Can you work these out from the model? Positions are in its coordinate system, mm. A direction names the side the tool comes from. Give positions to 0.01 mm unless a question says otherwise; leave off trailing zeros. Write each loop counter-clockwise with the first axis right and the second up, starting at its lowest first coordinate (ties: lowest second). Pieces come first, ordered by that corner, then holes. Notation, with made-up numbers: (-25.75, 10) - (15.25, 10) arc R22 cw to (15.25, 36) - close; hole circle Ø5 at (6, 24). An arc over 180 degrees is marked (long way). Return JSON: item names as keys, results as strings. Group by question number.
from build123d import *

# Parameters (mm, degrees)
F0_W      = 60
F0_H      = 60
F1_DEPTH  = 15
F2_W      = 25
F2_H      = 10
F3_DEPTH  = 150
F4_W      = 40
F4_H      = 40
F4_W_2    = 25
F4_H_2    = 10
F5_DEPTH  = 25
F6_SIZE2  = 39.99999
F6_SIZE   = 19.99999
F7_W      = 20
F7_H      = 5
F8_DEPTH  = 25
F9_R      = 3.5
F10_DEPTH = 150
F11_R     = 4
F12_DEPTH = 150


# Not quite as in the source:
# - a fillet or chamfer is up to 0.001 mm smaller than in the source, because OpenCascade refuses the exact size


with BuildPart() as f1:
    # F0 (on Top) → F1 (new body)
    with BuildSketch(Plane.XY):
        Rectangle(F0_W, F0_H)
    extrude(amount=F1_DEPTH)

    # F2 (on face) → F3 (join)
    with BuildSketch(Plane.XY.offset(15)):
        Rectangle(F2_W, F2_H)
    extrude(amount=F3_DEPTH)

    # F4 (on face) → F5 (join)
    with BuildSketch(Plane.XY.offset(165)):
        Rectangle(F4_W, F4_H)
        Rectangle(F4_W_2, F4_H_2, mode=Mode.SUBTRACT)
        Rectangle(F4_W_2, F4_H_2)
    extrude(amount=F5_DEPTH)

    # F6 (size 20 and 40 in the source; OpenCascade refuses exactly that, so slightly less here)
    f6_edges = [f1.edges().sort_by_distance(p)[0] for p in [
        (0, -20, 190),
    ]]
    f6_side = f1.faces().sort_by_distance((0, -20, 177.5))[0]
    chamfer(f6_edges, length=F6_SIZE, length2=F6_SIZE2, reference=f6_side)

    # F7 (on face) → F8 (cut)
    with BuildSketch(Plane.XZ.offset(5)):
        with Locations((0, 149.3448019028)):
            Rectangle(F7_W, F7_H)
    extrude(amount=-F8_DEPTH, mode=Mode.SUBTRACT)

    # F9 (on face) → F10 (join)
    with BuildSketch(Plane.YZ.offset(20)):
        with Locations((0, 172.1751581079)):
            Circle(F9_R)
    extrude(amount=F10_DEPTH)

    # F11 (on face) → F12 (join)
    with BuildSketch(Plane(origin=(-20, 0, 0), x_dir=(0, -1, 0), z_dir=(-1, 0, 0))):
        with Locations((0, 171.8452831515)):
            Circle(F11_R)
    extrude(amount=F12_DEPTH)


solid = f1.part
1) I need wall thicknesses on line 1 along X through (y, z) = (18.5, 174); line 2 along Y through (x, z) = (4.5, 99); line 3 along X through (y, z) = (-11.5, 14.5). Which ranges of each line are inside material? Lowest first, please.
2) Imagine slicing it at B-B, the plane y = -24.5. Write out the boundary of the cut face in (x, z).
3) On a 3-axis mill with a long thin cutter (end or side, diameter ignored), from which of +Z, -Z, +X, -X, +Y, -Y can I reach the whole of each face in a straight line? I mean faces 5 (the face through (-93.95, 0.87, 167.94)), 6 (the face through (0, 5, 89)), 7 (the face through (12.5, 0, 89)), 8 (the face through (0, -5, 89)). Say none if no direction works.
4) Imagine slicing it at C-C, the plane z = 139. Write out the boundary of the cut face in (x, y), and give its area (3 significant figures).
5) We'd pull the mould along X, two halves only. Please class faces 1 (the face through (0, 0, 0)), 2 (the face through (170, 0, 172)), 3 (the face through (0, 0, 151.845)), 4 (the face through (0, 0, 146.845)): pulls with the +X half, pulls with the -X half, needs draft (parallel to the pull), parting line crosses it, or undercut.
6) Imagine slicing it at A-A, the plane y = 0. Write out the boundary of the cut face in (x, z), and give its area (3 significant figures).
7) Will these pins go through, and if not, where does the flat tip stop? pin 1 Ø12.5 at (x, z) = (1, 77) entering from -Y; pin 2 Ø2.5 at (y, z) = (0.5, 150.5) entering from +X; pin 3 Ø1 at (x, y) = (-14, -22) entering from +Z; pin 4 Ø4 at (x, y) = (-10, 1.5) entering from -Z.
8) Imagine slicing it at D-D, the plane x = 97. Write out the boundary of the cut face in (y, z), and give its area (3 significant figures).
Resolved:
{
 "1": {"line 1": "-20 to 20", "line 2": "-5 to 5", "line 3": "-30 to 30"},
 "2": {"outline": "(-30, 0) - (30, 0) - (30, 15) - (-30, 15) - close"},
 "3": {"face 5": "-X", "face 6": "+X, -X, +Y", "face 7": "+X, +Y, -Y", "face 8": "+X, -X, -Y"},
 "4": {"outline": "(-12.5, -5) - (12.5, -5) - (12.5, 5) - (-12.5, 5) - close", "area": "250 mm^2"},
 "5": {"face 1": "needs draft", "face 2": "pulls with the +X half", "face 3": "undercut", "face 4": "undercut"},
 "6": {"outline": "(-170, 167.85) - (-20, 167.85) - (-20, 165) - (-12.5, 165) - (-12.5, 15) - (-30, 15) - (-30, 0) - (30, 0) - (30, 15) - (12.5, 15) - (12.5, 165) - (20, 165) - (20, 168.68) - (170, 168.68) - (170, 175.68) - (20, 175.68) - (20, 180) - (-20, 180) - (-20, 175.85) - (-170, 175.85) - close; hole (-10, 146.84) - (10, 146.84) - (10, 151.84) - (-10, 151.84) - close", "area": "7,400 mm^2"},
 "7": {"pin 1": "y = -5", "pin 2": "x = 12.5", "pin 3": "z = 15", "pin 4": "z = 0"},
 "8": {"outline": "circle Ø7 at (0, 172.18)", "area": "38.5 mm^2"}
}
